Verification items for the finished model (mm, model axes). Coordinates: 2 decimals unless noted, no trailing zeros. Order: outer loops, then holes, each group sorted by start corner. A loop starts at its lowest first (then second) coordinate and runs counter-clockwise, first axis right, second up. Notation, with made-up numbers: M -30,-29 L 23,-29 A28 cw 23,-6 Z; hole C -19,-28 d9. An arc over 180 degrees is marked long. Return JSON: item names as keys, results as strings.
```python
from build123d import *

# Parameters (mm, degrees)
PAD_DEPTH = 6.5


with BuildPart() as part:
    # Sketch → Pad (new body, symmetric)
    with BuildSketch(Plane.XZ):
        Polygon((0, 0), (150, 0), (150, 375), (90.992559, 375), (0, 125), align=None)
    extrude(amount=PAD_DEPTH, both=True)


solid = part.part
```
Q1. Go/stop test with a flat-tipped pin: pin 1 (1 mm diameter, centred on y = -5, z = 152.5, fed in from -X). Record where the tip stops, or that it passes through.
Values:
{"pin 1": "x = 9.83"}
Q2. Material ranges on line 1 along X through (y, z) = (1, 183.5); line 2 along X through (y, z) = (5.25, 178.5), recorded low to high.
Values:
{"line 1": "21.29 to 150", "line 2": "19.47 to 150"}
Q3. Cross-section at B-B, the plane z = 350. Record the boundary of the cut face in (x, y).
Values:
{"outline": "M 81.89,-6.5 L 150,-6.5 L 150,6.5 L 81.89,6.5 Z"}
Q4. Cross-section at C-C, the plane x = 67. Record the boundary of the cut face in (y, z).
Values:
{"outline": "M -6.5,0 L 6.5,0 L 6.5,309.08 L -6.5,309.08 Z"}
Q5. Cross-section at A-A, the plane y = -1.25. Record the boundary of the cut face in (x, z), and give its area (3 significant figures).
Values:
{"outline": "M 0,0 L 150,0 L 150,375 L 90.99,375 L 0,125 Z", "area": "44,900 mm^2"}
